from build123d import *

# Parameters (mm, degrees)
CUT_EXTRUDE1_DEPTH = 180.30421077


with BuildPart() as part:
    # Sketch1 → Revolve1 (revolve)
    with BuildSketch(Plane.XY, mode=Mode.PRIVATE) as revolve1_sk:
        Polygon((0, 15), (125, 15), (125, 10), (115, 0), (125, -10), (125, -15), (0, -15), align=None)
    revolve(revolve1_sk.sketch.rotate(Axis((0, -15, 0), (0, -1, 0)), 180), axis=Axis((0, -15, 0), (0, -1, 0)))

    # Sketch2 → Cut-Extrude1 (cut, through all)
    with BuildSketch(Plane(origin=(0, 15, 0), x_dir=(-1, 0, 0), z_dir=(0, 1, 0))):
        with BuildLine():
            Line((-5, 19.364916731), (-5, 25))
            Line((-5, 25), (5, 25))
            Line((5, 25), (5, 19.364916731))
            ThreePointArc((5, 19.364916731), (0, -20), (-5, 19.364916731))
        make_face()
    extrude(amount=-CUT_EXTRUDE1_DEPTH, mode=Mode.SUBTRACT)


solid = part.part
Can you work these out from the model? Positions are in its coordinate system, mm. A direction names the side the tool comes from. Round coordinates to 2 decimals unless told otherwise and drop trailing zeros. Order: outer loops, then holes, each group sorted by start corner. A loop starts at its lowest first (then second) coordinate and runs counter-clockwise, first axis right, second up. Notation, with made-up numbers: (-32, -17) - (-14, -17) arc R19 cw to (-14, 12) - close; hole circle Ø11 at (-12, 39.25). An arc over 180 degrees is marked (long way). Answer in a Markdown table with one row per item.
(1) Which directions (+Z, -Z, +X, -X, +Y, -Y) give clear straight access to the entire face, cutting with the end or side of a thin tool? Please do faces 1 (the face through (2, -15, 26)), 2 (the face through (25.04, 0.49, 112.74)), 3 (the face through (-5, 0, 22)).
From the geometry:
| item | result |
|---|---|
| face 1 | +Z, -Z, +X, -X, -Y |
| face 2 | none |
| face 3 | +Y, -Y |
(2) Suppose I cut it at A-A, the plane x = 0. Please give me the cut outline in (y, z), plus the area to 3 significant figures.
From the geometry:
| item | result |
|---|---|
| outline | (-15, -125) - (-10, -125) - (0, -115) - (10, -125) - (15, -125) - (15, -20) - (-15, -20) - close; (-15, 25) - (15, 25) - (15, 125) - (10, 125) - (0, 115) - (-10, 125) - (-15, 125) - close |
| area | 5,950 mm2 |
(3) Suppose I cut it at B-B, the plane z = 0. Please give me the cut outline in (x, y), plus the area to 3 significant figures.
From the geometry:
| item | result |
|---|---|
| outline | (-125, -15) - (-20, -15) - (-20, 15) - (-125, 15) - (-125, 10) - (-115, 0) - (-125, -10) - close; (20, -15) - (125, -15) - (125, -10) - (115, 0) - (125, 10) - (125, 15) - (20, 15) - close |
| area | 6,100 mm2 |
(4) For P1, Ø6, axis at y = 6.5, z = 21.5, coming from the -X side; P2, Ø1.5, axis at x = 86.5, y = -5.5, coming from the +Z side; P3, Ø12, axis at x = 66, y = -11, coming from the +Z side; P4, Ø24, axis at x = 0, z = 0, coming from the +Y side, each with a flat end and sliding along its axis, tell me the tip position at first contact or that it passes through.
From the geometry:
| item | result |
|---|---|
| P1 | stops at x = -122.67 |
| P2 | stops at z = 85.21 |
| P3 | stops at z = 109.66 |
| P4 | passes through |
(5) Please list where these lines run through material, in increasing order: L1, parallel to Y at x = 33, z = -112.5; L2, parallel to Z at x = -16, y = -11.5; L3, parallel to Y at x = -82.5, z = 87. Write a range as from..to.
From the geometry:
| item | result |
|---|---|
| L1 | y = -15..-2.24, 2.24..15 |
| L2 | z = -123.97..-12, 12..123.97 |
| L3 | y = -15..-4.9, 4.9..15 |
(6) If we mould it in two halves opening along Y, with no side actions, what happens to faces 4 (the face through (-2, 15, 26)), 5 (the face through (-62.16, -0.63, -97.5)), 6 (the face through (5, 0, 22))? For each: released by +Y, released by -Y, zero draft, split by the parting line, or undercut.
From the geometry:
| item | result |
|---|---|
| face 4 | released by +Y |
| face 5 | undercut |
| face 6 | zero draft |
(7) Suppose I cut it at C-C, the plane y = -3.25. Please give me the cut outline in (x, z), plus the area to 3 significant figures.
From the geometry:
| item | result |
|---|---|
| outline | circle Ø236.5 at (0, 0); hole (-5, 19.36) arc R20 ccw (long way) to (5, 19.36) - (5, 25) - (-5, 25) - close |
| area | 42,600 mm2 |
